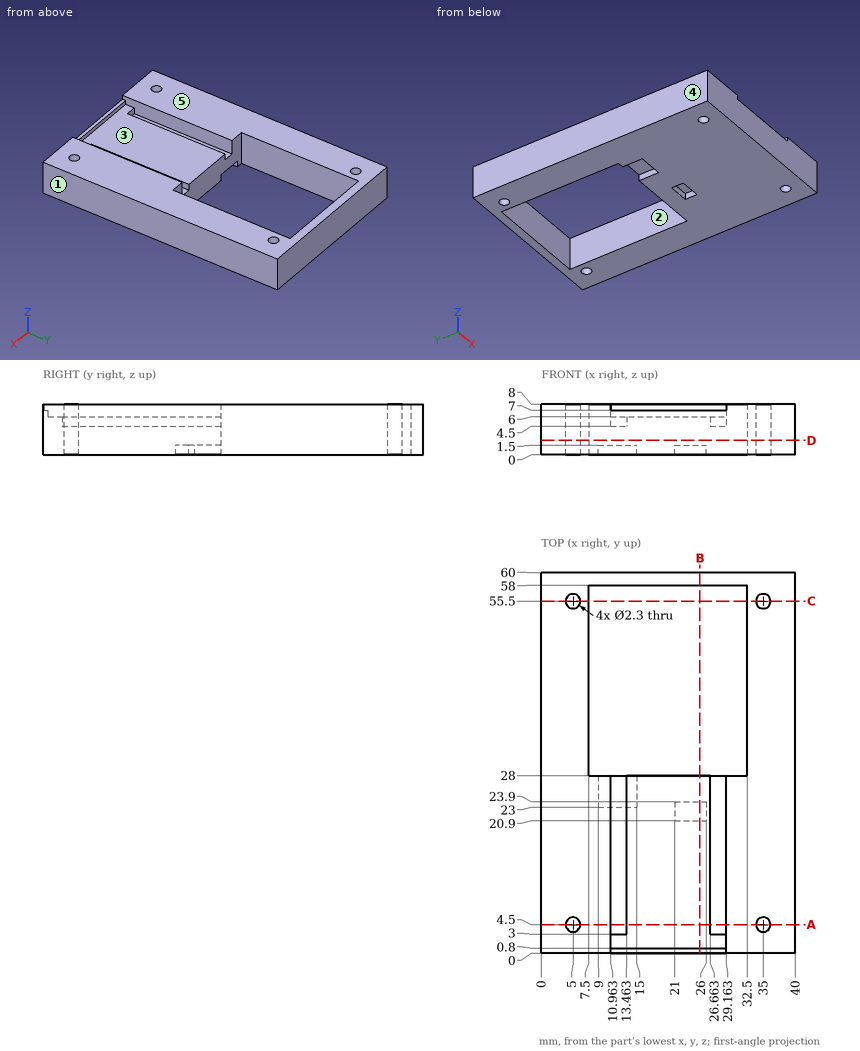
Can you work these out from the drawing? Everything is in mm from the part's minimum corner. A direction names the side the tool comes from. Give positions to 0.01 mm unless a question says otherwise; leave off trailing zeros. Order: outer loops, then holes, each group sorted by start corner. A loop starts at its lowest first (then second) coordinate and runs counter-clockwise, first axis right, second up. Notation, with made-up numbers: M 44,39 L 94,39 A18 cw 94,55 Z; hole C 59,-12 d3. An arc over 180 degrees is marked long. One line per question, with ' | ' between items.
1. For the marked faces 1 and 2, which set-ups out of +Z, -Z, +X, -X, +Y, -Y let a thin tool reach every point of the face, with its end or its side?
Results:
face 1: +Z, -Z, +X, +Y, -Y | face 2: +Z, -Z
2. I'm going to push flat-ended pins straight in: pin 1 (2.5 mm diameter, centred on x = 22.5, y = 22.5, fed in from -Z); pin 2 (3 mm diameter, centred on x = 27.5, y = 19, fed in from +Z); pin 3 (0.8 mm diameter, centred on x = 12, y = 20.5, fed in from +Z). Where does each tip first touch, or does it pass through?
Results:
pin 1: z = 1.5 | pin 2: z = 6 | pin 3: z = 4.5
3. If I drill on line 1 (Y direction, x = 5, z = 5.25); line 2 (X direction, y = 54, z = 4.5); line 3 (Y direction, x = 25, z = 0.5), over which ranges is the centre line in solid material (lowest first)?
Results:
line 1: 0 to 3.35, 5.65 to 54.35, 56.65 to 60 | line 2: 0 to 7.5, 32.5 to 40 | line 3: 0 to 20.9, 23.9 to 28, 58 to 60
4. I want a section at D-D (z = 2.25). List the corners of the cut face in (x, y) for me.
Results:
outline: M 0,0 L 40,0 L 40,60 L 0,60 Z; hole C 5,4.5 d2.3; hole C 5,55.5 d2.3; hole M 7.5,28 L 32.5,28 L 32.5,58 L 7.5,58 Z; hole C 35,4.5 d2.3; hole C 35,55.5 d2.3
5. I want a section at C-C (y = 55.5). List the corners of the cut face in (x, z) for me.
Results:
outline: M 0,0 L 3.85,0 L 3.85,8 L 0,8 Z; M 6.15,0 L 7.5,0 L 7.5,8 L 6.15,8 Z; M 32.5,0 L 33.85,0 L 33.85,8 L 32.5,8 Z; M 36.15,0 L 40,0 L 40,8 L 36.15,8 Z
6. I want a section at B-B (x = 25). List the corners of the cut face in (y, z) for me, and give its area (3 significant figures).
Results:
outline: M 0,0 L 20.9,0 L 20.9,1.5 L 23.9,1.5 L 23.9,0 L 28,0 L 28,6 L 0.8,6 L 0.8,7 L 0,7 Z; M 58,0 L 60,0 L 60,8 L 58,8 Z | area: 180 mm²
7. I want a section at A-A (y = 4.5). List the corners of the cut face in (x, z) for me, and give its area (3 significant figures).
Results:
outline: M 0,0 L 3.85,0 L 3.85,8 L 0,8 Z; M 6.15,0 L 33.85,0 L 33.85,8 L 29.16,8 L 29.16,4.5 L 26.66,4.5 L 26.66,6 L 13.46,6 L 13.46,4.5 L 10.96,4.5 L 10.96,8 L 6.15,8 Z; M 36.15,0 L 40,0 L 40,8 L 36.15,8 Z | area: 239 mm²
8. We'd pull the mould along X, two halves only. Please class the marked faces 3, 4 and 5: +X half, -X half, draft (parallel to the pull), parting line (faces both ways), or undercut.
Results:
face 3: undercut | face 4: -X half | face 5: draft
